Read the model definition and answer for the solid it produces. Units are mm, in the model's axes. A direction names the side the tool comes from. Give positions to 0.01 mm unless a question says otherwise; leave off trailing zeros. Loops run counter-clockwise (first coordinate to the right, second up) from the corner with the lowest first, then second, coordinate; pieces in that order, holes last. Notation, with made-up numbers: (26.5, -37.5) -> (57.5, -37.5) arc R18 ccw to (57.5, -5.5) -> close; hole circle Ø10 at (51, -19.5). An arc over 180 degrees is marked (long way). Return JSON: item names as keys, results as strings. Group by question number.
from build123d import *

# Parameters (mm, degrees)
SKETCH1_R           = 36.5
BOSS_EXTRUDE1_DEPTH = 42.5
SKETCH2_W           = 73
SKETCH2_H           = 44
BOSS_EXTRUDE2_DEPTH = 42.5
SKETCH3_R           = 31.5
CUT_EXTRUDE1_DEPTH  = 39.5
SKETCH4_W           = 63
SKETCH4_H           = 41.5
CUT_EXTRUDE2_DEPTH  = 39.5
SKETCH5_R           = 5
SKETCH5_R_2         = 1.45
CUT_EXTRUDE3_DEPTH  = 3


with BuildPart() as part:
    # Sketch1 → Boss-Extrude1 (new body)
    with BuildSketch(Plane.XY.offset(350)):
        with Locations((300, 300)):
            Circle(SKETCH1_R)
    extrude(amount=BOSS_EXTRUDE1_DEPTH)

    # Sketch2 → Boss-Extrude2 (add)
    with BuildSketch(Plane.XY.offset(350)):
        with Locations((300, 322)):
            Rectangle(SKETCH2_W, SKETCH2_H)
    extrude(amount=BOSS_EXTRUDE2_DEPTH)

    # Sketch3 → Cut-Extrude1 (cut)
    with BuildSketch(Plane.XY.offset(350)):
        with Locations((300, 300)):
            Circle(SKETCH3_R)
    extrude(amount=CUT_EXTRUDE1_DEPTH, mode=Mode.SUBTRACT)

    # Sketch4 → Cut-Extrude2 (cut)
    with BuildSketch(Plane.XY.offset(350)):
        with Locations((300, 320.75)):
            Rectangle(SKETCH4_W, SKETCH4_H)
    extrude(amount=CUT_EXTRUDE2_DEPTH, mode=Mode.SUBTRACT)

    # Sketch5 → Cut-Extrude3 (cut)
    with BuildSketch(Plane.XY.offset(389.5)):
        with Locations((300, 300)):
            Circle(SKETCH5_R)
        with Locations((286.774831823, 318.202882373)):
            Circle(SKETCH5_R_2)
        with Locations((278.601228383, 293.047117627)):
            Circle(SKETCH5_R_2)
        with Locations((300, 277.5)):
            Circle(SKETCH5_R_2)
        with Locations((321.398771617, 293.047117627)):
            Circle(SKETCH5_R_2)
        with Locations((313.225168177, 318.202882373)):
            Circle(SKETCH5_R_2)
    extrude(amount=CUT_EXTRUDE3_DEPTH, mode=Mode.SUBTRACT)


solid = part.part
1. Straight lines are drawn through the part: line 1 (Y direction, x = 300, z = 390.4); line 2 (X direction, y = 332.5, z = 376.5); line 3 (X direction, y = 300, z = 390). For each, find the intervals that lie inside material, in ascending order. Write a range as from..to.
2. Section B-B on z = 366.5 is taken. Determine the outline of the cut face in (x, y).
3. Section A-A on y = 277.5 is taken. Determine the outline of the cut face in (x, z), then the cut area to 3 significant figures.
4. Flat-ended cylindrical pins translate along their axes: pin 1 Ø3.5 at (x, y) = (286.77, 318.2) entering from -Z; pin 2 Ø2.5 at (x, y) = (313.23, 318.2) entering from +Z; pin 3 Ø2 at (y, z) = (289, 364.5) entering from -X; pin 4 Ø5 at (x, z) = (300, 378) entering from -Y. Find the tip coordinate at first contact, or state that the pin passes through.
5. Section C-C on x = 300 is taken. Determine the outline of the cut face in (y, z), then the cut area to 3 significant figures.
6. Which of the six approach directions +Z, -Z, +X, -X, +Y, -Y give full straight-line access (tool end or side, diameter ignored) to faces 5 (the flat face through (267, 301, 350)), 6 (the flat face through (268.5, 320, 369))?
7. Section D-D on y = 331 is taken. Determine the outline of the cut face in (x, z).
8. Determine the mould class of faces 1 (the cylindrical face through (312.074, 317.321, 390.979)), 2 (the flat face through (299, 344, 371)), 3 (the flat face through (336.5, 322, 371)), 4 (the cylindrical face through (299.2, 263.51, 370.95)) for opening direction Y: pulls with the +Y half, pulls with the -Y half, needs draft (parallel to the pull), parting line crosses it, or undercut.
Completed:
{
 "1": {"line 1": "y = 263.5..276.05, 278.95..295, 305..344", "line 2": "x = 263.5..268.5, 331.5..336.5", "line 3": "x = 263.5..295, 305..336.5"},
 "2": {"outline": "(263.5, 300) arc R36.5 ccw to (336.5, 300) -> (336.5, 344) -> (263.5, 344) -> close; hole (268.5, 300) arc R31.5 ccw to (331.5, 300) -> (331.5, 341.5) -> (268.5, 341.5) -> close"},
 "3": {"outline": "(271.26, 350) -> (277.95, 350) -> (277.95, 389.5) -> (298.55, 389.5) -> (298.55, 392.5) -> (271.26, 392.5) -> close; (301.45, 389.5) -> (322.05, 389.5) -> (322.05, 350) -> (328.74, 350) -> (328.74, 392.5) -> (301.45, 392.5) -> close", "area": "693 mm²"},
 "4": {"pin 1": "stops at z = 389.5", "pin 2": "passes through", "pin 3": "stops at x = 264.9", "pin 4": "stops at y = 263.5"},
 "5": {"outline": "(263.5, 350) -> (268.5, 350) -> (268.5, 389.5) -> (276.05, 389.5) -> (276.05, 392.5) -> (263.5, 392.5) -> close; (278.95, 389.5) -> (295, 389.5) -> (295, 392.5) -> (278.95, 392.5) -> close; (305, 389.5) -> (341.5, 389.5) -> (341.5, 350) -> (344, 350) -> (344, 392.5) -> (305, 392.5) -> close", "area": "499 mm²"},
 "6": {"face 5": "-Z, +X, -X, +Y, -Y", "face 6": "-Z"},
 "7": {"outline": "(263.5, 350) -> (268.5, 350) -> (268.5, 389.5) -> (331.5, 389.5) -> (331.5, 350) -> (336.5, 350) -> (336.5, 392.5) -> (263.5, 392.5) -> close"},
 "8": {"face 1": "undercut", "face 2": "pulls with the +Y half", "face 3": "needs draft", "face 4": "pulls with the -Y half"}
}
